```python
from build123d import *

# Parameters (mm, degrees)
SKETCH3_R                    = 57.5
SKETCH3_R_2                  = 22.5
BOSS_EXTRUDE2_DEPTH          = 7
SKETCH12_R                   = 11.01
CUT_EXTRUDE7_DEPTH           = 82.618012718
CHAMFER5_SIZE                = 0.5
CIRPATTERN4_COUNT            = 4
CHAMFER5_OF_CIRPATTERN4_SIZE = 0.5


with BuildPart() as part:
    # Sketch3 → Boss-Extrude2 (new body)
    with BuildSketch(Plane(origin=(0, 0, 0), x_dir=(-1, 0, 0), z_dir=(0, 0, -1))):
        Circle(SKETCH3_R)
        Circle(SKETCH3_R_2, mode=Mode.SUBTRACT)
    extrude(amount=BOSS_EXTRUDE2_DEPTH)

    # Sketch12 → Cut-Extrude7 (cut, through all)
    with BuildSketch(Plane.XY):
        with Locations((-40, 0)):
            Circle(SKETCH12_R)
    cut_extrude7 = extrude(amount=-CUT_EXTRUDE7_DEPTH, mode=Mode.SUBTRACT)

    # Chamfer5
    chamfer5_edges = [part.edges().sort_by_distance(p)[0] for p in [
        (-51.01, 0, -7),
        (-51.01, 0, 0),
    ]]
    chamfer(chamfer5_edges, length=CHAMFER5_SIZE)

    # CirPattern4: Cut-Extrude7 ×4 about axis
    cirpattern4_axis = Axis((0, 0, 0), (0, 0, 1))
    for i in range(1, CIRPATTERN4_COUNT):
        add(cut_extrude7.rotate(cirpattern4_axis, i * 360 / CIRPATTERN4_COUNT), mode=Mode.SUBTRACT)

    # Chamfer5 of CirPattern4
    chamfer5_of_cirpattern4_edges = [part.edges().sort_by_distance(p)[0] for p in [
        (0, -51.01, -7),
        (0, -51.01, 0),
        (51.01, 0, -7),
        (51.01, 0, 0),
        (0, 51.01, -7),
        (0, 51.01, 0),
    ]]
    chamfer(chamfer5_of_cirpattern4_edges, length=CHAMFER5_OF_CIRPATTERN4_SIZE)


solid = part.part
```
Source: CAD feature listing. Evaluate the final solid. Frame: model axes, mm. Coordinates: 2 decimals unless noted, no trailing zeros. Order: outer loops, then holes, each group sorted by start corner. A loop starts at its lowest first (then second) coordinate and runs counter-clockwise, first axis right, second up. Notation, with made-up numbers: (29, 86) - (50, 86) arc R29 cw to (50, 116) - close; hole circle Ø11 at (69, 16). An arc over 180 degrees is marked (long way). One line per item, written item: value.
1) Cut plane D-D on y = -40. Output: boundary loops of the cut face in (x, z).
Computed values:
outline: (-41.31, -7) - (-11.51, -7) - (-11.01, -6.5) - (-11.01, -0.5) - (-11.51, 0) - (-41.31, 0) - close; (11.01, -6.5) - (11.51, -7) - (41.31, -7) - (41.31, 0) - (11.51, 0) - (11.01, -0.5) - close
2) Ray query, line 1 (Y direction, x = 0.5, z = -3.25); line 2 (X direction, y = -10, z = -5); line 3 (Y direction, x = -4.5, z = -6.5). Return the intervals inside material, ascending. Write a range as [from, to].
Computed values:
line 1: y = [-57.5, -51], [-29, -22.49], [22.49, 29], [51, 57.5]
line 2: x = [-56.62, -44.61], [-35.39, -20.16], [20.16, 35.39], [44.61, 56.62]
line 3: y = [-57.32, -50.05], [-29.95, -22.05], [22.05, 29.95], [50.05, 57.32]
3) Cut plane C-C on z = -2.5. Output: boundary loops of the cut face in (x, y), plus the area to 3 significant figures.
Computed values:
outline: circle Ø115 at (0, 0); hole circle Ø22.02 at (-40, 0); hole circle Ø45 at (0, 0); hole circle Ø22.02 at (0, -40); hole circle Ø22.02 at (0, 40); hole circle Ø22.02 at (40, 0)
area: 7,270 mm^2
4) Mould query, pull axis Y, two halves, no side actions, for faces 1 (the face through (12.465, -56.133, -3.451)), 2 (the face through (6.699, -48.737, -3.458)), 3 (the face through (-25, 1, -7)). Classes: released by +Y, released by -Y, zero draft, split by the parting line, or undercut.
Computed values:
face 1: split by the parting line
face 2: undercut
face 3: zero draft
5) Cut plane A-A on y = 0. Output: boundary loops of the cut face in (x, z), plus the area to 3 significant figures.
Computed values:
outline: (-57.5, -7) - (-51.51, -7) - (-51.01, -6.5) - (-51.01, -0.5) - (-51.51, 0) - (-57.5, 0) - close; (-28.99, -6.5) - (-28.49, -7) - (-22.5, -7) - (-22.5, 0) - (-28.49, 0) - (-28.99, -0.5) - close; (22.5, -7) - (28.49, -7) - (28.99, -6.5) - (28.99, -0.5) - (28.49, 0) - (22.5, 0) - close; (51.01, -6.5) - (51.51, -7) - (57.5, -7) - (57.5, 0) - (51.51, 0) - (51.01, -0.5) - close
area: 181 mm^2
6) Cut plane B-B on x = 15. Output: boundary loops of the cut face in (y, z).
Computed values:
outline: (-55.51, -7) - (-16.77, -7) - (-16.77, 0) - (-55.51, 0) - close; (16.77, -7) - (55.51, -7) - (55.51, 0) - (16.77, 0) - close
